Geometry: final body of the model. Coordinates: model frame, mm. Coordinates: 2 decimals unless noted, no trailing zeros. Order: outer loops, then holes, each group sorted by start corner. A loop starts at its lowest first (then second) coordinate and runs counter-clockwise, first axis right, second up. Notation, with made-up numbers: (82, 55.25) -> (107, 55.25) arc R20 ccw to (107, 73.25) -> close; hole circle Ø2 at (27, 58.25). An arc over 180 degrees is marked (long way). Use one line per item in the form item = value.
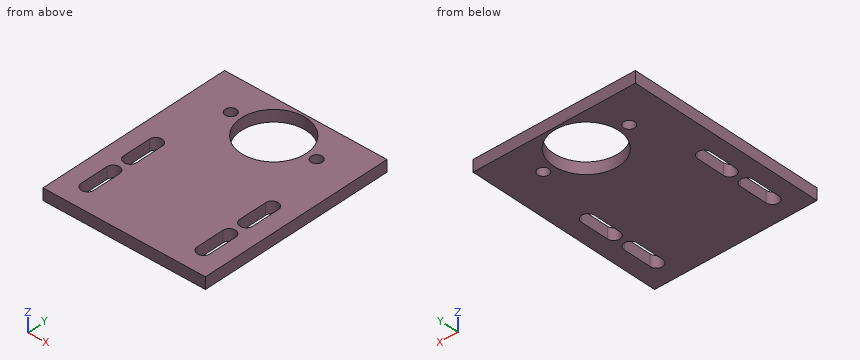
```python
from build123d import *

# Parameters (mm, degrees)
SKETCH1_R           = 2.4
SKETCH1_R_2         = 14
BOSS_EXTRUDE1_DEPTH = 5


with BuildPart() as part:
    # Sketch1 → Boss-Extrude1 (new body)
    with BuildSketch(Plane.XY):
        Polygon((-35, 50), (-35, -15), (-35, -35), (35, -35), (35, -15), (35, 50), align=None)
        with BuildLine():
            ThreePointArc((-22.25, -25), (-25, -27.75), (-27.75, -25))
            Line((-27.75, -25), (-27.75, -13))
            ThreePointArc((-27.75, -13), (-25, -10.25), (-22.25, -13))
            Line((-22.25, -13), (-22.25, -25))
        make_face(mode=Mode.SUBTRACT)
        with BuildLine():
            ThreePointArc((-22.25, -5), (-25, -7.75), (-27.75, -5))
            Line((-27.75, -5), (-27.75, 7))
            ThreePointArc((-27.75, 7), (-25, 9.75), (-22.25, 7))
            Line((-22.25, 7), (-22.25, -5))
        make_face(mode=Mode.SUBTRACT)
        with BuildLine():
            Line((27.75, -13), (27.75, -25))
            ThreePointArc((27.75, -25), (25, -27.75), (22.25, -25))
            Line((22.25, -25), (22.25, -13))
            ThreePointArc((22.25, -13), (25, -10.25), (27.75, -13))
        make_face(mode=Mode.SUBTRACT)
        with BuildLine():
            Line((27.75, 7), (27.75, -5))
            ThreePointArc((27.75, -5), (25, -7.75), (22.25, -5))
            Line((22.25, -5), (22.25, 7))
            ThreePointArc((22.25, 7), (25, 9.75), (27.75, 7))
        make_face(mode=Mode.SUBTRACT)
        with Locations((-18.5, 35)):
            Circle(SKETCH1_R, mode=Mode.SUBTRACT)
        with Locations((0, 35)):
            Circle(SKETCH1_R_2, mode=Mode.SUBTRACT)
        with Locations((18.5, 35)):
            Circle(SKETCH1_R, mode=Mode.SUBTRACT)
    extrude(amount=BOSS_EXTRUDE1_DEPTH)


solid = part.part
```
1) Section D-D, the plane x = -25. Output: boundary loops of the cut face in (y, z), and give its area (3 significant figures).
Results found:
outline = (-35, 0) -> (-27.75, 0) -> (-27.75, 5) -> (-35, 5) -> close; (-10.25, 0) -> (-7.75, 0) -> (-7.75, 5) -> (-10.25, 5) -> close; (9.75, 0) -> (50, 0) -> (50, 5) -> (9.75, 5) -> close
area = 250 mm2
2) Section B-B, the plane y = 6. Output: boundary loops of the cut face in (x, z).
Results found:
outline = (-35, 0) -> (-27.75, 0) -> (-27.75, 5) -> (-35, 5) -> close; (-22.25, 0) -> (22.25, 0) -> (22.25, 5) -> (-22.25, 5) -> close; (27.75, 0) -> (35, 0) -> (35, 5) -> (27.75, 5) -> close
3) Contact query for a flat-ended pin moving along its axis: P1, Ø4, axis at x = -18.5, y = 35, coming from the -Z side. Output: stop coordinate, or through.
Results found:
P1 = through
4) Section C-C, the plane z = 0.75. Output: boundary loops of the cut face in (x, y), and give its area (3 significant figures).
Results found:
outline = (-35, -35) -> (35, -35) -> (35, 50) -> (-35, 50) -> close; hole (-27.75, -25) arc R2.75 ccw to (-22.25, -25) -> (-22.25, -13) arc R2.75 ccw to (-27.75, -13) -> close; hole (-27.75, -5) arc R2.75 ccw to (-22.25, -5) -> (-22.25, 7) arc R2.75 ccw to (-27.75, 7) -> close; hole circle Ø4.8 at (-18.5, 35); hole circle Ø28 at (0, 35); hole circle Ø4.8 at (18.5, 35); hole (22.25, -25) arc R2.75 ccw to (27.75, -25) -> (27.75, -13) arc R2.75 ccw to (22.25, -13) -> close; hole (22.25, -5) arc R2.75 ccw to (27.75, -5) -> (27.75, 7) arc R2.75 ccw to (22.25, 7) -> close
area = 4,940 mm2
5) Section A-A, the plane y = 35. Output: boundary loops of the cut face in (x, z), and give its area (3 significant figures).
Results found:
outline = (-35, 0) -> (-20.9, 0) -> (-20.9, 5) -> (-35, 5) -> close; (-16.1, 0) -> (-14, 0) -> (-14, 5) -> (-16.1, 5) -> close; (14, 0) -> (16.1, 0) -> (16.1, 5) -> (14, 5) -> close; (20.9, 0) -> (35, 0) -> (35, 5) -> (20.9, 5) -> close
area = 162 mm2
6) Material intervals for probe 1 along X at (y, z) = (-5, 4.1); probe 2 along Y at (x, z) = (0, 2.5); probe 3 along Y at (x, z) = (18.5, 3.9), sorted ascending. Write a range as from..to.
Results found:
probe_1 = -35..-27.75, -22.25..22.25, 27.75..35
probe_2 = -35..21, 49..50
probe_3 = -35..32.6, 37.4..50
